Can you work these out from the model? Positions are in its coordinate system, mm. Face numbers are marked on the shaded views. A direction names the side the tool comes from. Give positions to 0.01 mm unless a question says otherwise; leave off trailing zeros. Loops run counter-clockwise (first coordinate to the right, second up) from the corner with the lowest first, then second, coordinate; pieces in that order, holes last. Notation, with made-up numbers: (71, 82.25) - (79, 82.25) arc R14 ccw to (79, 108.25) - close; hole circle Ø8 at (50, 69). An arc over 180 degrees is marked (long way). Use a Markdown table: item, result. Add a question column.
```python
from build123d import *

# Parameters (mm, degrees)
SALIENTE_EXTRUIR1_DEPTH = 80
CROQUIS2_R              = 25
SALIENTE_EXTRUIR2_DEPTH = 30
SALIENTE_EXTRUIR3_START = 30
CROQUIS3_R              = 25
SALIENTE_EXTRUIR3_DEPTH = 30
CROQUIS4_R              = 20
SALIENTE_EXTRUIR5_DEPTH = 20
SALIENTE_EXTRUIR6_START = -20
CROQUIS5_R              = 20
SALIENTE_EXTRUIR6_DEPTH = 20


with BuildPart() as part:
    # Croquis1 → Saliente-Extruir1 (new body)
    with BuildSketch(Plane.XY):
        Polygon((0, 0), (40, 0), (40, 70), (-40, 70), (-40, 0), align=None)
    extrude(amount=-SALIENTE_EXTRUIR1_DEPTH)

    # Croquis2 → Saliente-Extruir2 (add)
    with BuildSketch(Plane(origin=(40, 0, 0), x_dir=(0, 0, -1), z_dir=(1, 0, 0))):
        with Locations((40, 35)):
            Circle(CROQUIS2_R)
    extrude(amount=SALIENTE_EXTRUIR2_DEPTH)

    # Croquis3 → Saliente-Extruir3 (add)
    with BuildSketch(Plane.ZY.offset(40).offset(SALIENTE_EXTRUIR3_START)):
        with Locations(Location((-40, 35, 0), (0, 0, 180))):
            Circle(CROQUIS3_R)
    extrude(amount=-SALIENTE_EXTRUIR3_DEPTH)

    # Croquis4 → Saliente-Extruir5 (add)
    with BuildSketch(Plane.XY.offset(-10)):
        with BuildLine():
            Line((-40, 110), (-40, 70))
            Line((-40, 70), (0, 70))
            Line((0, 70), (40, 70))
            Line((40, 70), (40, 110))
            ThreePointArc((40, 110), (0, 150), (-40, 110))
        make_face()
        with Locations((0, 110)):
            Circle(CROQUIS4_R, mode=Mode.SUBTRACT)
    extrude(amount=-SALIENTE_EXTRUIR5_DEPTH)

    # Croquis5 → Saliente-Extruir6 (add)
    with BuildSketch(Plane(origin=(0, 0, -70), x_dir=(-1, 0, 0), z_dir=(0, 0, -1)).offset(SALIENTE_EXTRUIR6_START)):
        with BuildLine():
            Line((-40, 110), (-40, 70))
            Line((-40, 70), (40, 70))
            Line((40, 70), (40, 110))
            ThreePointArc((40, 110), (0, 150), (-40, 110))
        make_face()
        with Locations(Location((0, 110, 0), (0, 0, 180))):
            Circle(CROQUIS5_R, mode=Mode.SUBTRACT)
    extrude(amount=SALIENTE_EXTRUIR6_DEPTH)


solid = part.part
```
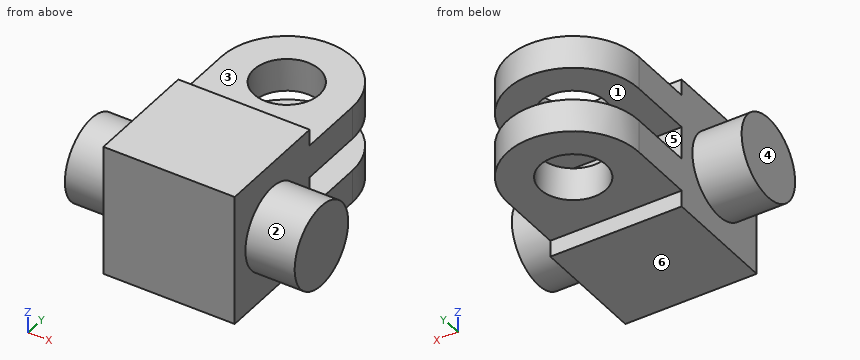
1. Please list where these lines run through material, in increasing order: line 1 along Z through (x, y) = (15.5, 126.5); line 2 along X through (y, z) = (110, -54.75); line 3 along Y through (x, z) = (0, -20). Write a range as [from, to].
2. Suppose I cut it at A-A (x = 0). List the corners of the cut face in (y, z) for me.
3. If we mould it in two halves opening along Z, with no side actions, what happens to the marked faces 4, 5 and 6? For each: released by +Z, released by -Z, zero draft, split by the parting line, or undercut.
4. Will these pins go through, and if not, where does the flat tip stop? P1, Ø2, axis at x = -14.5, z = -66.5, coming from the +Y side; P2, Ø24, axis at x = 18, y = 100, coming from the +Z side; P3, Ø3, axis at y = 104.5, z = -19, coming from the +X side; P4, Ø12, axis at x = 19.5, y = 73, coming from the +Z side.
5. Suppose I cut it at D-D (y = 132). List the corners of the cut face in (x, z) for me, and give its area (3 significant figures).
6. Suppose I cut it at C-C (y = 35). List the corners of the cut face in (x, z) for me.
7. On a 3-axis mill with a long thin cutter (end or side, diameter ignored), from which of +Z, -Z, +X, -X, +Y, -Y can I reach the whole of each face in a straight line? I mean the marked faces 1, 2 and 3. Say none if no direction works.
8. Suppose I cut it at B-B (z = -54). List the corners of the cut face in (x, y) for me.
Results below:
| question | item | result |
|---|---|---|
| 1 | line 1 | [-70, -50], [-30, -10] |
| 1 | line 2 | [-40, -20], [20, 40] |
| 1 | line 3 | [0, 90], [130, 150] |
| 2 | outline | (0, -80) - (70, -80) - (70, -70) - (90, -70) - (90, -50) - (70, -50) - (70, -30) - (90, -30) - (90, -10) - (70, -10) - (70, 0) - (0, 0) - close; (130, -70) - (150, -70) - (150, -50) - (130, -50) - close; (130, -30) - (150, -30) - (150, -10) - (130, -10) - close |
| 3 | face 4 | zero draft |
| 3 | face 5 | undercut |
| 3 | face 6 | released by -Z |
| 4 | P1 | y = 147.65 |
| 4 | P2 | z = -10 |
| 4 | P3 | x = 40 |
| 4 | P4 | z = 0 |
| 5 | outline | (-33.41, -70) - (33.41, -70) - (33.41, -50) - (-33.41, -50) - close; (-33.41, -30) - (33.41, -30) - (33.41, -10) - (-33.41, -10) - close |
| 5 | area | 2,670 mm² |
| 6 | outline | (-70, -65) - (-40, -65) - (-40, -80) - (40, -80) - (40, -65) - (70, -65) - (70, -15) - (40, -15) - (40, 0) - (-40, 0) - (-40, -15) - (-70, -15) - close |
| 7 | face 1 | +X, -X, +Y |
| 7 | face 2 | +X |
| 7 | face 3 | +Z, +X, -X, +Y |
| 8 | outline | (-70, 14.29) - (-40, 14.29) - (-40, 0) - (40, 0) - (40, 14.29) - (70, 14.29) - (70, 55.71) - (40, 55.71) - (40, 110) arc R40 ccw to (-40, 110) - (-40, 55.71) - (-70, 55.71) - close; hole circle Ø40 at (0, 110) |
